```python
from build123d import *

# Parameters (mm, degrees)
F0_W      = 1308.1
F0_H      = 501.65
F1_DEPTH  = 812.8
F2_W      = 1428.75
F2_H      = 527.05
F3_DEPTH  = 63.5
F4_SIZE2  = 50.79999
F4_SIZE   = 25.39999
F5_W      = 1428.75
F5_H      = 527.05
F5_H_2    = 254
F6_DEPTH  = 38.1
F7_R      = 19.05
F8_W      = 355.6
F8_H      = 558.8
F9_DEPTH  = 482.6
F10_W     = 457.2
F10_H     = 558.8
F11_DEPTH = 152.4
F13_DEPTH = 50.8


# Not quite as in the source:
# - a fillet or chamfer is up to 0.001 mm smaller than in the source, because OpenCascade refuses the exact size


with BuildPart() as f1:
    # F0 (on Top) → F1 (new body)
    with BuildSketch(Plane.XY):
        with Locations((-654.05, 250.825)):
            Rectangle(F0_W, F0_H)
    extrude(amount=F1_DEPTH)

    # F2 (on face) → F3 (join)
    with BuildSketch(Plane.XY.offset(812.8)):
        with Locations((-654.05, 238.125)):
            Rectangle(F2_W, F2_H)
    extrude(amount=F3_DEPTH)

    # F4 (size 25.4 and 50.8 in the source; OpenCascade refuses exactly that, so slightly less here)
    f4_edges = [f1.edges().sort_by_distance(p)[0] for p in [
        (-1368.425, 238.125, 812.8),
        (-654.05, -25.4, 812.8),
        (60.325, 238.125, 812.8),
    ]]
    f4_side = f1.faces().sort_by_distance((-654.05, -10.171381, 812.8))[0]
    chamfer(f4_edges, length=F4_SIZE, length2=F4_SIZE2, reference=f4_side)

    # F5 (on face) → F6 (join)
    with BuildSketch(Plane.XY.offset(876.3)):
        with Locations((-654.05, 238.125)):
            Rectangle(F5_W, F5_H)
        with Locations((-654.05, 628.65)):
            Rectangle(F5_W, F5_H_2)
    extrude(amount=F6_DEPTH)

    # F7
    f7_edges = [f1.edges().sort_by_distance(p)[0] for p in [
        (-1368.425, 365.125, 914.4),
        (-654.05, -25.4, 914.4),
        (60.325, 365.125, 914.4),
    ]]
    fillet(f7_edges, radius=F7_R)

    # F8 (on face) → F9 (cut)
    with BuildSketch(Plane.XZ):
        with Locations((-279.4, 431.8)):
            Rectangle(F8_W, F8_H)
        with Locations((-736.6, 431.8)):
            Rectangle(F8_W, F8_H)
    extrude(amount=-F9_DEPTH, mode=Mode.SUBTRACT)

    # F10 (on face) → F11 (cut)
    with BuildSketch(Plane.YZ.offset(-457.2)):
        with Locations((254, 431.8)):
            Rectangle(F10_W, F10_H)
    extrude(amount=-F11_DEPTH, mode=Mode.SUBTRACT)

    # F12 (on face) → F13 (cut)
    with BuildSketch(Plane.XY.offset(152.4)):
        Polygon((-101.6, 482.6), (-914.4, 482.6), (-914.4, 25.4), (-558.8, 25.4), (-457.2, 25.4), (-101.6, 25.4), align=None)
    extrude(amount=-F13_DEPTH, mode=Mode.SUBTRACT)


solid = f1.part
```
The listing builds one solid part. Answer for the finished solid, in the listing's coordinates (mm). A direction names the side the tool comes from. Coordinates: 2 decimals unless noted, no trailing zeros. Loops run counter-clockwise (first coordinate to the right, second up) from the corner with the lowest first, then second, coordinate; pieces in that order, holes last. Notation, with made-up numbers: (54.25, 82) -> (106.25, 82) arc R17 cw to (106.25, 109) -> close; hole circle Ø5 at (-18.75, 73.5). An arc over 180 degrees is marked (long way). Return JSON: item names as keys, results as strings. Group by question number.
(1) Determine the mould class of faces 5 (the flat face through (-664.1, -12.9, 838.6)), 6 (the flat face through (-514, 257, 101.6)), 7 (the flat face through (-664, 755.65, 895)), 8 (the flat face through (-664, 630, 876.3)) for opening direction Y: released by +Y, released by -Y, zero draft, split by the parting line, or undercut.
(2) Find the intervals of material crossed by probe 1 along Z at (x, y) = (-123, 212.5); probe 2 along X at (y, z) = (325, 268); probe 3 along Y at (x, z) = (-362.5, 134), in increasing order. Write a range as from..to.
(3) A cutting plane is placed at D-D on y = 574. Write down the section's boundary in (x, z) (3 decimals).
(4) Given pin 1 Ø1 at (y, z) = (135, 99.5) entering from -X; pin 2 Ø12.5 at (y, z) = (6.5, 463.5) entering from +X; pin 3 Ø1 at (x, y) = (-887.5, 652) entering from -Z, each flat-ended and moving along its own axis, determine where each tip first touches the part or whether it passes through.
(5) A cutting plane is placed at B-B on y = 148. Write down the section's boundary in (x, z) (3 decimals), and give its area (3 significant figures).
(6) Which of the six approach directions +Z, -Z, +X, -X, +Y, -Y give full straight-line access (tool end or side, diameter ignored) to faces 1 (the flat face through (-664, 501.65, 432)), 2 (the flat face through (-514, 482.6, 411)), 3 (the flat face through (-518, 0, 401)), 4 (the flat face through (6, 252, 812.8))?
(7) A cutting plane is placed at A-A on z = 216. Write down the section's boundary in (x, y).
The answers:
{
 "1": {"face 5": "released by -Y", "face 6": "undercut", "face 7": "released by +Y", "face 8": "zero draft"},
 "2": {"probe 1": "z = 0..101.6, 711.2..914.4", "probe 2": "x = -1308.1..-914.4, -101.6..0", "probe 3": "y = 0..25.4, 482.6..501.65"},
 "3": {"outline": "(-1368.425, 876.3) -> (60.325, 876.3) -> (60.325, 895.35) arc R19.05 ccw to (41.275, 914.4) -> (-1349.375, 914.4) arc R19.05 ccw to (-1368.425, 895.35) -> close"},
 "4": {"pin 1": "stops at x = -1308.1", "pin 2": "stops at x = 0", "pin 3": "stops at z = 876.3"},
 "5": {"outline": "(-1368.425, 863.6) -> (-1343.025, 812.8) -> (-1308.1, 812.8) -> (-1308.1, 0) -> (0, 0) -> (0, 812.8) -> (34.925, 812.8) -> (60.325, 863.6) -> (60.325, 895.35) arc R19.05 ccw to (41.275, 914.4) -> (-1349.375, 914.4) arc R19.05 ccw to (-1368.425, 895.35) -> close; hole (-914.4, 101.6) -> (-101.6, 101.6) -> (-101.6, 711.2) -> (-914.4, 711.2) -> close", "area": "711,000 mm^2"},
 "6": {"face 1": "-Z, +X, -X, +Y", "face 2": "none", "face 3": "-Z, +X, -X, -Y", "face 4": "-Z, +X, +Y, -Y"},
 "7": {"outline": "(-1308.1, 0) -> (-914.4, 0) -> (-914.4, 482.6) -> (-101.6, 482.6) -> (-101.6, 0) -> (0, 0) -> (0, 501.65) -> (-1308.1, 501.65) -> close; (-558.8, 0) -> (-457.2, 0) -> (-457.2, 25.4) -> (-558.8, 25.4) -> close"}
}
